Autodesk Inventor part; units mm, degrees
ref_plane "YZ Plane" through (0, 0, 0) normal (1, 0, 0) x (0, 1, 0)
ref_plane "XZ Plane" through (0, 0, 0) normal (0, 1, 0) x (-1, 0, 0)
ref_plane "XY Plane" through (0, 0, 0) normal (0, 0, 1) x (1, 0, 0)
sketch "Skizze2" plane through (0, 0, 0) normal (1, 0, 0) x (0, 1, 0)
  line L0 (33.2284, 9.1468) -> (33.2284, 6.5468)
  line L1 (33.2284, 9.1468) -> (33.2284, 15.4468)
  line L2 (33.2284, 15.4468) -> (42.7284, 15.4468)
  line L3 (41.2284, 6.5468) -> (33.2284, 6.5468)
  line L4 (42.7284, 14.2468) -> (41.2284, 14.2468)
  line L5 (42.7284, 14.2468) -> (42.7284, 15.4468)
  line L6 (33.2284, 15.4468) -> (42.7284, 15.4468)
  line L7 (33.2284, 9.1468) -> (33.2284, 15.4468)
  line L8 (33.2284, 9.1468) -> (41.2284, 9.1468)
  line L9 (41.2284, 14.2468) -> (41.2284, 9.1468)
  line L10 (42.7284, 14.2468) -> (42.7284, 15.4468)
  line L11 (41.2284, 9.1468) -> (41.2284, 6.5468)
  point P0 (0, 0)
extrude "Extrusion1" add sketch "Skizze2" along normal blind 69.4
sketch "Skizze3" plane through (0, 0, 0) normal (-1, 0, 0) x (0, 0, 1)
  line L0 (14.2468, 42.7284) -> (14.2468, 41.2284)
  line L1 (14.2468, 42.7284) -> (15.4468, 42.7284)
  line L2 (15.4468, 33.2284) -> (15.4468, 42.7284)
  line L3 (9.1468, 33.2284) -> (15.4468, 33.2284)
  line L4 (9.1468, 33.2284) -> (9.1468, 41.2284)
  line L5 (14.2468, 41.2284) -> (9.1468, 41.2284)
  line L6 (6.5468, 33.2284) -> (6.5468, 41.2284)
  line L7 (6.5468, 41.2284) -> (9.1468, 41.2284)
  line L8 (9.1468, 41.2284) -> (9.1468, 33.2284)
  line L9 (9.1468, 33.2284) -> (6.5468, 33.2284)
  line L10 (6.5468, 33.2284) -> (6.5468, 41.2284)
  point P0 (0, 0)
extrude "Extrusion2" cut sketch "Skizze3" against normal blind 10 contours L4 L9 L6 L7
sketch "Skizze4" plane through (0, 33.2284, 15.4468) normal (0, 0, 1) x (1, 0, 0)
  line L0 (0, 0) -> (10, 0) construction
  line L1 (5, 0) -> (5, 9.5) construction
  line L2 (0, 9.5) -> (69.4, 9.5) construction
  circle A0 centre (5, 4) radius 3
  line L3 (0, 9.5) -> (0, 0) construction
  point P0 (0, -33.2284)
  dimension "d4" = 6
  dimension "d5" = 5
  dimension "d6" = 4
extrude "Extrusion3" cut sketch "Skizze4" against normal blind 3.4
sketch "Skizze5" plane through (5, 37.2284, 12.0468) normal (0, 0, 1) x (1, 0, 0)
  circle A0 centre (0, 0) radius 3
  circle A1 centre (0, 0) radius 1.75
  point P0 (-5, -37.2284)
  dimension "d9" = 3.5
extrude "Extrusion4" cut sketch "Skizze5" against normal blind 3.4 contours A1
mirror "Spiegeln1" about plane through (69.4, 37.2284, 7.8468) normal (1, 0, 0) of "Extrusion4", "Extrusion3", "Extrusion2", "Extrusion1"
properties part number "Case_bottom_front"
Could you check a few things on this model? Use its own coordinates, in mm. A direction names the side the tool comes from. Round coordinates to 2 decimals unless told otherwise and drop trailing zeros. Loops run counter-clockwise (first coordinate to the right, second up) from the corner with the lowest first, then second, coordinate; pieces in that order, holes last.
Q1. For P1, Ø4, axis at x = 135, y = 37.5, coming from the -Z side; P2, Ø3, axis at x = 5, y = 37.23, coming from the -Z side; P3, Ø3, axis at x = 69.5, z = 10.5, coming from the +Y side; P4, Ø0.8, axis at y = 36, z = 8, coming from the -X side, each with a flat end and sliding along its axis, tell me the tip position at first contact or that it passes through.
Q2. On a 3-axis mill with a long thin cutter (end or side, diameter ignored), from which of +Z, -Z, +X, -X, +Y, -Y can I reach the whole of each face in a straight line? I mean faces 4 (the cylindrical face through (131.03, 38.38, 13.77)), 5 (the flat face through (133, 39, 9.147)), 6 (the flat face through (5, 35, 9.147)), 7 (the flat face through (68, 41.228, 10)). Say none if no direction works.
Q3. I want a section at A-A (x = 5). Write out the boundary of the cut face in (y, z).
Q4. Please list where these lines run through material, in increasing order: L1, parallel to Y at x = 5, z = 14.2; L2, parallel to X at y = 36.5, z = 15; L3, parallel to X at y = 37.25, z = 10.75.
Q5. Thinking about a two-plate mould opening in X: for faces 1 (the flat face through (0, 38, 12)), 2 (the cylindrical face through (4.62, 35.52, 10.62)), 3 (the flat face through (68, 33.228, 11)), which applies, pulls with the +X half, pulls with the -X half, needs draft (parallel to the pull), parting line crosses it, or undercut?
Answer below:
1. P1: stops at z = 9.15
1. P2: passes through
1. P3: stops at y = 41.23
1. P4: stops at x = 10
2. face 4: +Z
2. face 5: -Z, +X, +Y, -Y
2. face 6: -Z, -X, +Y, -Y
2. face 7: -Z, +X, -X, +Y
3. outline: (33.23, 9.15) - (35.48, 9.15) - (35.48, 12.05) - (34.23, 12.05) - (34.23, 15.45) - (33.23, 15.45) - close; (38.98, 9.15) - (41.23, 9.15) - (41.23, 14.25) - (42.73, 14.25) - (42.73, 15.45) - (40.23, 15.45) - (40.23, 12.05) - (38.98, 12.05) - close
4. L1: y = 33.23 to 34.23, 40.23 to 41.23
4. L2: x = 0 to 2.09, 7.91 to 130.89, 136.71 to 138.8
4. L3: x = 0 to 3.25, 6.75 to 132.05, 135.55 to 138.8
5. face 1: pulls with the -X half
5. face 2: undercut
5. face 3: needs draft
